```python
from build123d import *

# Parameters (mm, degrees)
PADS_SKETCH_R   = 5.42
PADS_DEPTH      = 2.03
PADS_2_DEPTH    = 2.03
PADS_3_DEPTH    = 2.03
PADS_4_DEPTH    = 2.03
PADS_SKETCH_R_2 = 9
PADS_5_DEPTH    = 2.03
CONNECTOR_DEPTH = 2.03


with BuildPart() as part:
    # Pads Sketch → Pads (new body)
    with BuildSketch(Plane.XY):
        with Locations((-10.069761866, -34.302512969)):
            Circle(PADS_SKETCH_R)
    extrude(amount=PADS_DEPTH)



with BuildPart() as body_2:
    # Pads Sketch → Pads 2 (new body)
    with BuildSketch(Plane.XY):
        with Locations((-27.013589298, -23.416415038)):
            Circle(PADS_SKETCH_R)
    extrude(amount=PADS_2_DEPTH)


with BuildPart() as body_3:
    # Pads Sketch → Pads 3 (new body)
    with BuildSketch(Plane.XY):
        with Locations((-32.525938452, 14.836638023)):
            Circle(PADS_SKETCH_R)
    extrude(amount=PADS_3_DEPTH)


with BuildPart() as body_4:
    # Pads Sketch → Pads 4 (new body)
    with BuildSketch(Plane.XY):
        with Locations((-19.345084764, 30.063768817)):
            Circle(PADS_SKETCH_R)
    extrude(amount=PADS_4_DEPTH)


with BuildPart() as body_5:
    # Pads Sketch → Pads 5 (new body)
    with BuildSketch(Plane.XY):
        with Locations((-35.384500255, -5.09898438)):
            Circle(PADS_SKETCH_R_2)
    extrude(amount=PADS_5_DEPTH)


with BuildPart() as part_1:
    add(part.part)

    add(body_2.part)  # Connector merges body 2

    add(body_3.part)  # Connector merges body 3

    add(body_4.part)  # Connector merges body 4

    add(body_5.part)  # Connector merges body 5
    # Connector Sketch → Connector (add)
    with BuildSketch(Plane.XY.offset(2.03)):
        with BuildLine():
            Line((-24.578173622, 28.652676688), (-22.176010765, 25.44183654))
            ThreePointArc((-22.176010765, 25.44183654), (-33.404947793, -4.813726513), (-14.090471833, -30.667916517))
            Line((-14.090471833, -30.667916517), (-15.488346946, -34.426350502))
            ThreePointArc((-15.488346946, -34.426350502), (-37.364052717, -5.384242247), (-24.578173622, 28.652676688))
        make_face()
    extrude(amount=-CONNECTOR_DEPTH)


solid = part_1.part
```
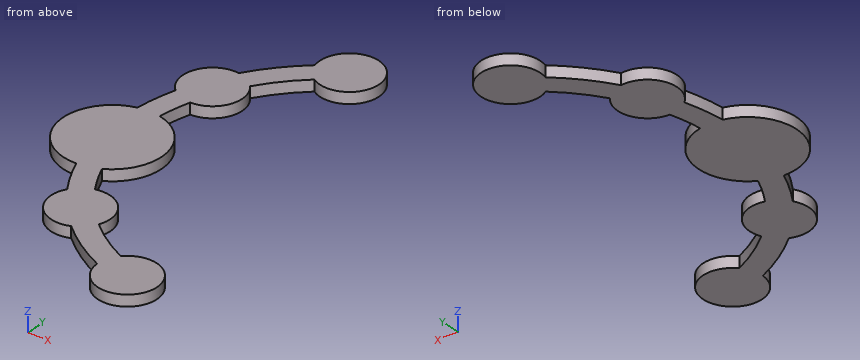
The listing builds one solid part. Answer for the finished solid, in the listing's coordinates (mm). Coordinates: 2 decimals unless noted, no trailing zeros. Write each loop counter-clockwise with the first axis right and the second up, starting at its lowest first coordinate (ties: lowest second). Pieces come first, ordered by that corner, then holes. Notation, with made-up numbers: (-9, -33) - (15, -33) arc R36 cw to (15, 5) - close; hole circle Ø4 at (79.5, 57.5). An arc over 180 degrees is marked (long way). One line per item, written item: value.
1) Find section D-D (x = -11.5). Give the vertices of the cut face in (y, z), and give its area (3 significant figures).
Geometry check:
outline: (-39.53, 0) - (-29.07, 0) - (-29.07, 2.03) - (-39.53, 2.03) - close
area: 21.2 mm2
2) Consider line 1 along Y through (x, z) = (-29, 0.75); line 2 along X through (y, z) = (15, 1.5); line 3 along Y through (x, z) = (-20.5, 1.7). Determine where each line is inside the solid, lowest interval first. Write a range as from..to.
Geometry check:
line 1: y = -28.46..-17.26, -11.44..1.24, 10.72..24.17
line 2: x = -37.94..-27.11
line 3: y = -31.7..-26.81, 24.77..35.36
3) Find section C-C (y = 5). Give the vertices of the cut face in (x, z).
Geometry check:
outline: (-37.42, 0) - (-33.38, 0) - (-33.38, 2.03) - (-37.42, 2.03) - close
4) Find section A-A (z = 1.3). Give the vertices of the cut face in (x, y), and give its area (3 significant figures).
Geometry check:
outline: (-37.58, 3.63) arc R9 ccw to (-35.02, -14.09) arc R37.75 ccw to (-31.64, -20.59) arc R5.42 ccw to (-24.87, -28.4) arc R37.75 ccw to (-15.49, -34.43) arc R5.42 ccw (long way) to (-14.09, -30.67) arc R33.75 cw to (-22.04, -25.56) arc R5.42 ccw to (-28.43, -18.19) arc R33.75 cw to (-31.13, -13.03) arc R9 ccw to (-33.55, 3.71) arc R33.75 cw to (-32.41, 9.42) arc R5.42 ccw to (-28.36, 18.3) arc R33.75 cw to (-22.18, 25.44) arc R5.42 ccw (long way) to (-24.58, 28.65) arc R37.75 ccw to (-31.88, 20.22) arc R5.42 ccw to (-36.17, 10.82) arc R37.75 ccw to start
area: 752 mm2
5) Find section B-B (x = -19). Give the vertices of the cut face in (y, z), and give its area (3 significant figures).
Geometry check:
outline: (-32.62, 0) - (-27.89, 0) - (-27.89, 2.03) - (-32.62, 2.03) - close; (24.65, 0) - (35.47, 0) - (35.47, 2.03) - (24.65, 2.03) - close
area: 31.6 mm2
